Verification items for the finished model (mm, model axes). A direction names the side the tool comes from. Give positions to 0.01 mm unless a question says otherwise; leave off trailing zeros. Write each loop counter-clockwise with the first axis right and the second up, starting at its lowest first coordinate (ties: lowest second). Pieces come first, ordered by that corner, then holes. Notation, with made-up numbers: (-15, 37.25) - (16, 37.25) arc R26 ccw to (16, 70.25) - close; hole circle Ø8 at (87.25, 10.25). An arc over 180 degrees is marked (long way). Put each result on its own line as item: value.
from build123d import *

# Parameters (mm, degrees)
F0_W     = 406.4
F0_H     = 152.4
F1_DEPTH = 19.05
F2_W     = 6.35
F2_H     = 6.35
F3_DEPTH = 152.401
F4_R     = 44.45
F5_DEPTH = 19.051
F6_R     = 50.8
F6_R_2   = 44.45
F7_DEPTH = 63.5


with BuildPart() as f1:
    # F0 (on Top) → F1 (new body)
    with BuildSketch(Plane.XY):
        Rectangle(F0_W, F0_H)
    extrude(amount=F1_DEPTH)

    # F2 (on face) → F3 (cut, through all)
    with BuildSketch(Plane.XZ.offset(76.2)):
        Polygon((-203.2, 9.525), (-203.2, 0), (-184.15, 0), (-184.15, 6.35), (-184.15, 9.525), align=None)
        Polygon((184.15, 6.35), (184.15, 0), (203.2, 0), (203.2, 9.525), (184.15, 9.525), align=None)
        with Locations((180.975, 3.175)):
            Rectangle(F2_W, F2_H)
    extrude(amount=-F3_DEPTH, mode=Mode.SUBTRACT)

    # F4 (on face) → F5 (cut, through all)
    with BuildSketch(Plane(origin=(0, 0, 0), x_dir=(1, 0, 0), z_dir=(0, 0, -1))):
        with Locations((-127, 0)):
            Circle(F4_R)
    extrude(amount=-F5_DEPTH, mode=Mode.SUBTRACT)

    # F6 (on face) → F7 (join)
    with BuildSketch(Plane.XY.offset(19.05)):
        with Locations((-127, 0)):
            Circle(F6_R)
        with Locations((-127, 0)):
            Circle(F6_R_2, mode=Mode.SUBTRACT)
    extrude(amount=F7_DEPTH)


solid = f1.part
Q1. Section check C-C, the plane y = -36. Record the cut outline in (x, z) (3 decimals), plus the area to 3 significant figures.
Answers follow:
outline: (-203.2, 9.525) - (-184.15, 9.525) - (-184.15, 0) - (-153.073, 0) - (-153.073, 82.55) - (-162.842, 82.55) - (-162.842, 19.05) - (-203.2, 19.05) - close; (-100.927, 0) - (177.8, 0) - (177.8, 6.35) - (184.15, 6.35) - (184.15, 9.525) - (203.2, 9.525) - (203.2, 19.05) - (-91.158, 19.05) - (-91.158, 82.55) - (-100.927, 82.55) - close
area: 7,590 mm2
Q2. Section check A-A, the plane y = 0. Record the cut outline in (x, z) (3 decimals).
Answers follow:
outline: (-203.2, 9.525) - (-184.15, 9.525) - (-184.15, 0) - (-171.45, 0) - (-171.45, 82.55) - (-177.8, 82.55) - (-177.8, 19.05) - (-203.2, 19.05) - close; (-82.55, 0) - (177.8, 0) - (177.8, 6.35) - (184.15, 6.35) - (184.15, 9.525) - (203.2, 9.525) - (203.2, 19.05) - (-76.2, 19.05) - (-76.2, 82.55) - (-82.55, 82.55) - close
Q3. Section check D-D, the plane z = 33.5. Record the cut outline in (x, y), plus the area to 3 significant figures.
Answers follow:
outline: circle Ø101.6 at (-127, 0); hole circle Ø88.9 at (-127, 0)
area: 1,900 mm2
Q4. Section check B-B, the plane x = -127. Record the cut outline in (y, z), plus the area to 3 significant figures.
Answers follow:
outline: (-76.2, 0) - (-44.45, 0) - (-44.45, 82.55) - (-50.8, 82.55) - (-50.8, 19.05) - (-76.2, 19.05) - close; (44.45, 0) - (76.2, 0) - (76.2, 19.05) - (50.8, 19.05) - (50.8, 82.55) - (44.45, 82.55) - close
area: 2,020 mm2
Q5. Go/stop test with flat-tipped pins: pin 1 Ø8 at (x, y) = (-74, -41.5) entering from -Z; pin 2 Ø5.5 at (x, y) = (-194.5, 13.5) entering from -Z (3 decimals); pin 3 Ø1.5 at (x, y) = (61.5, 56) entering from +Z; pin 4 Ø8 at (y, z) = (40.5, 57) entering from -X. Record where each tip stops, or that it passes through.
Answers follow:
pin 1: stops at z = 0
pin 2: stops at z = 9.525
pin 3: stops at z = 19.05
pin 4: stops at x = -162.33
Q6. Set-up check for faces 4 (the face through (-184.15, -1, 5)), 5 (the face through (-167.313, -30.911, 50.356)), 6 (the face through (194, -1, 9.525)): record each of +Z, -Z, +X, -X, +Y, -Y from which the full face is reachable in a straight line by a thin tool's end or side.
Answers follow:
face 4: -Z, -X, +Y, -Y
face 5: +Z
face 6: -Z, +X, +Y, -Y
Q7. Scan lines: line 1 along Y through (x, z) = (-127, 31.5); line 2 along Z through (x, y) = (-41.5, -53.5); line 3 along X through (y, z) = (-2.5, 34.5). Record each from-to range of solid material in increasing order.
Answers follow:
line 1: y = -50.8 to -44.45, 44.45 to 50.8
line 2: z = 0 to 19.05
line 3: x = -177.74 to -171.38, -82.62 to -76.26
Q8. Release check for a two-part mould opening along X. For faces 1 (the face through (-3, -76.2, 9)), 2 (the face through (203.2, -1, 14)), 3 (the face through (-84.603, 13.352, 40.697)) record: released by +X, released by -X, zero draft, split by the parting line, or undercut.
Answers follow:
face 1: zero draft
face 2: released by +X
face 3: undercut
